from build123d import *

# Parameters (mm, degrees)
SKETCH1_W           = 101
SKETCH1_H           = 8
SKETCH1_W_2         = 99
SKETCH1_H_2         = 6
BOSS_EXTRUDE1_DEPTH = 10
SKETCH2_R           = 1.2
BOSS_EXTRUDE2_DEPTH = 2
SKETCH3_W           = 103
SKETCH3_H           = 10
SKETCH3_W_2         = 101
SKETCH3_H_2         = 8
BOSS_EXTRUDE3_DEPTH = 6
FILLET4_R           = 1
FILLET5_R           = 1
FILLET6_R           = 1
FILLET7_R           = 1
FILLET8_R           = 0.5
FILLET9_R           = 0.5


# Some blends are built 0.0001 mm under size
with BuildPart() as part:
    # Sketch1 → Boss-Extrude1 (new body)
    with BuildSketch(Plane(origin=(0, 0, 0), x_dir=(1, 0, 0), z_dir=(0, 1, 0))):
        Rectangle(SKETCH1_W, SKETCH1_H)
        Rectangle(SKETCH1_W_2, SKETCH1_H_2, mode=Mode.SUBTRACT)
    extrude(amount=BOSS_EXTRUDE1_DEPTH)

    # Sketch2 → Boss-Extrude2 (add)
    # profile 1 of 3: a face of its own
    with BuildSketch(Plane.XZ):
        with BuildLine():
            Line((48, 4), (50.5, 4))
            Line((50.5, 4), (50.5, 13))
            ThreePointArc((50.5, 13), (46.232233047, 14.767766953), (48, 10.5))
            Line((48, 10.5), (48, 4))
        make_face()
        with Locations(Location((48, 13, 0), (0, 0, 270))):
            Circle(SKETCH2_R, mode=Mode.SUBTRACT)
    # profile 2 of 3: a face of its own
    with BuildSketch(Plane.XZ):
        with BuildLine():
            Line((48, -4), (50.5, -4))
            Line((50.5, -4), (50.5, -11))
            ThreePointArc((50.5, -11), (46.232233047, -12.767766953), (48, -8.5))
            Line((48, -8.5), (48, -4))
        make_face()
        with Locations(Location((48, -11, 0), (0, 0, 270))):
            Circle(SKETCH2_R, mode=Mode.SUBTRACT)
    # profile 3 of 3: a face of its own
    with BuildSketch(Plane.XZ):
        with BuildLine():
            Line((-66.4, 15), (-48.835058433, 15))
            Line((-48.835058433, 15), (-48.835058433, 4))
            Line((-48.835058433, 4), (-50.5, 4))
            Line((-50.5, 4), (-50.5, -4))
            Line((-50.5, -4), (-51.901659191, -4))
            Line((-51.901659191, -4), (-51.901659191, 11))
            Line((-51.901659191, 11), (-66.4, 11))
            ThreePointArc((-66.4, 11), (-68.4, 13), (-66.4, 15))
        make_face()
        with Locations(Location((-66.4, 13, 0), (0, 0, 270))):
            Circle(SKETCH2_R, mode=Mode.SUBTRACT)
    extrude(amount=-BOSS_EXTRUDE2_DEPTH)

    # Sketch3 → Boss-Extrude3 (add)
    with BuildSketch(Plane(origin=(0, 10, 0), x_dir=(1, 0, 0), z_dir=(0, 1, 0))):
        Rectangle(SKETCH3_W, SKETCH3_H)
        Rectangle(SKETCH3_W_2, SKETCH3_H_2, mode=Mode.SUBTRACT)
    extrude(amount=-BOSS_EXTRUDE3_DEPTH)

    # Fillet4
    fillet4_edges = [part.edges().sort_by_distance(p)[0] for p in [
        (0, 4, -4),
    ]]
    fillet(fillet4_edges, radius=FILLET4_R - 0.0001)  # a hair under: the kernel refuses the full size

    # Fillet5
    fillet5_edges = [part.edges().sort_by_distance(p)[0] for p in [
        (0, 4, 4),
    ]]
    fillet(fillet5_edges, radius=FILLET5_R - 0.0001)  # a hair under: the kernel refuses the full size

    # Fillet6
    fillet6_edges = [part.edges().sort_by_distance(p)[0] for p in [
        (50.5, 4, 0),
    ]]
    fillet(fillet6_edges, radius=FILLET6_R - 0.0001)  # a hair under: the kernel refuses the full size

    # Fillet7
    fillet7_edges = [part.edges().sort_by_distance(p)[0] for p in [
        (-50.5, 4, 0),
    ]]
    fillet(fillet7_edges, radius=FILLET7_R - 0.0001)  # a hair under: the kernel refuses the full size

    # Fillet8
    fillet8_edges = [part.edges().sort_by_distance(p)[0] for p in [
        (-51.901659191, 1, 11),
        (-48.835058433, 1, 15),
    ]]
    fillet(fillet8_edges, radius=FILLET8_R)

    # Fillet9
    # the kernel refuses this fillet: 0.5 mm, written as the material it takes off along each edge
    with BuildSketch(Plane(origin=(51.5, 11.25, -5), x_dir=(-1, 0, 0), z_dir=(0, -1, 0))) as fillet9_piece_1:
        with BuildLine():
            CenterArc((FILLET9_R, -FILLET9_R), FILLET9_R, 90, 90)
            Line((0, -FILLET9_R), (0, 0))
            Line((0, 0), (FILLET9_R, 0))
        make_face()
    extrude(amount=8.5, mode=Mode.SUBTRACT)
    with BuildSketch(Plane(origin=(51.5, 11.25, 5), x_dir=(-1, 0, 0), z_dir=(0, -1, 0)), Plane(origin=(-51.5, 11.25, 5), x_dir=(0, 0, -1), z_dir=(0, -1, 0)), Plane(origin=(-51.5, 11.25, -5), x_dir=(1, 0, 0), z_dir=(0, -1, 0))) as fillet9_piece_2:
        with BuildLine():
            CenterArc((FILLET9_R, FILLET9_R), FILLET9_R, 180, 90)
            Line((0, FILLET9_R), (0, 0))
            Line((0, 0), (FILLET9_R, 0))
        make_face()
    extrude(amount=8.5, mode=Mode.SUBTRACT)


solid = part.part
For this review, take the finished solid that the model builds, in its own axes (mm). A direction names the side the tool comes from. Coordinates: 2 decimals unless noted, no trailing zeros. Order: outer loops, then holes, each group sorted by start corner. A loop starts at its lowest first (then second) coordinate and runs counter-clockwise, first axis right, second up. Notation, with made-up numbers: (26, 50) -> (60, 50) arc R23 cw to (60, 76) -> close; hole circle Ø7 at (40.25, 27). An arc over 180 degrees is marked (long way). Return JSON: item names as keys, results as strings.
1. For line 1 (X direction, y = 0.8, z = 13); line 2 (Z direction, x = -66.4, y = 1.4); line 3 (Z direction, x = -8.5, y = 4.25), list the stretches that pass through material, from the lowest coordinate up. Write a range as from..to.
Answer block:
{"line 1": "-68.4..-67.6, -65.2..-48.84, 45.5..46.8, 49.2..50.5", "line 2": "11..11.8, 14.2..15", "line 3": "-5..-3, 3..5"}
2. The part is to be moulded in two halves that separate along Z. For faces 5 (the flat face through (-49.5, 5, 0)), 6 (the flat face through (-1, 7, 5)), 7 (the cylindrical face through (-68.4, 1, 13)), say which applies: +Z half, -Z half, draft (parallel to the pull), parting line (faces both ways), or undercut.
Answer block:
{"face 5": "undercut", "face 6": "+Z half", "face 7": "parting line"}
3. Machinability: for faces 1 (the flat face through (-51.902, 1, 3)), 2 (the flat face through (48, 1, -6)), 3 (the flat face through (50.5, 1, 1)), 4 (the flat face through (49.5, 5, 0)), which of the approach directions +Z, -Z, +X, -X, +Y, -Y give a long, thin tool a straight path to every point of the face, cutting with its end or side? Answer none if there is none.
Answer block:
{"face 1": "-Z, -X, +Y, -Y", "face 2": "-X, -Y", "face 3": "+Z, -Z, +X, -Y", "face 4": "+Y, -Y"}
4. For pin 1 Ø1.6 at (x, y) = (-58, 1.5) entering from +Z; pin 2 Ø1.5 at (x, y) = (14.5, 1.5) entering from +Z; pin 3 Ø5 at (y, z) = (2.5, -0.5) entering from -X; pin 4 Ø2 at (x, z) = (-66.4, 13) entering from -Y, all flat-tipped, find the tip position at first contact; note any pin that passes through.
Answer block:
{"pin 1": "z = 15", "pin 2": "z = 4", "pin 3": "x = -51.9", "pin 4": "through"}
5. We need section B-B on z = 7.5. Write out the cut boundary in (x, y).
Answer block:
{"outline": "(-51.9, 0) -> (-48.84, 0) -> (-48.84, 2) -> (-51.9, 2) -> close; (48, 0) -> (50.5, 0) -> (50.5, 2) -> (48, 2) -> close"}
6. We need section D-D on x = -60. Write out the cut boundary in (y, z).
Answer block:
{"outline": "(0, 11) -> (2, 11) -> (2, 15) -> (0, 15) -> close"}
7. We need section C-C on y = 7. Write out the cut boundary in (x, z).
Answer block:
{"outline": "(-51.5, -4.5) arc R0.5 ccw to (-51, -5) -> (51, -5) arc R0.5 ccw to (51.5, -4.5) -> (51.5, 4.5) arc R0.5 ccw to (51, 5) -> (-51, 5) arc R0.5 ccw to (-51.5, 4.5) -> close; hole (-49.5, -3) -> (49.5, -3) -> (49.5, 3) -> (-49.5, 3) -> close"}
